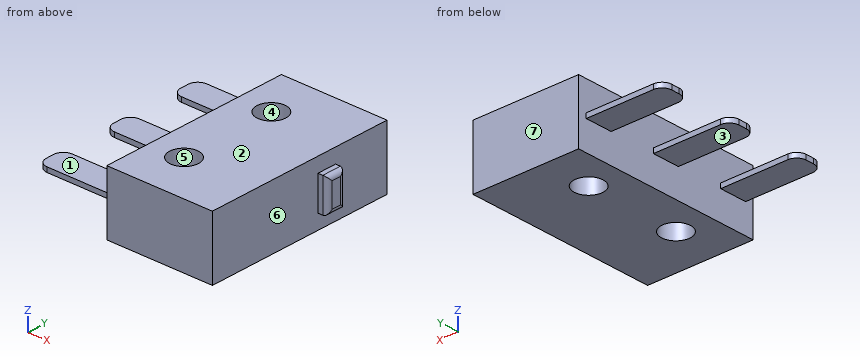
```python
from build123d import *

# Parameters (mm, degrees)
SKETCH_W     = 11
SKETCH_H     = 20
PAD_DEPTH    = 6.5
SKETCH001_W  = 2.85
SKETCH001_H  = 0.5
PAD001_DEPTH = 8
FILLET_R     = 1
SKETCH002_W  = 2
SKETCH002_H  = 3.5
PAD002_DEPTH = 1
FILLET001_R  = 0.5
SKETCH003_R  = 1.5
POCKET_DEPTH = 6.501


with BuildPart() as part:
    # Sketch → Pad (new body)
    with BuildSketch(Plane.XY):
        Rectangle(SKETCH_W, SKETCH_H)
    extrude(amount=PAD_DEPTH)

    # Sketch001 → Pad001 (new body)
    with BuildSketch(Plane(origin=(-5.5, 0, 0), x_dir=(0, -1, 0), z_dir=(-1, 0, 0))):
        with Locations((-7.7, 3.25)):
            Rectangle(SKETCH001_W, SKETCH001_H)
        with Locations((0, 3.25)):
            Rectangle(SKETCH001_W, SKETCH001_H)
        with Locations((7.7, 3.25)):
            Rectangle(SKETCH001_W, SKETCH001_H)
    extrude(amount=PAD001_DEPTH)

    # Fillet
    fillet_edges = [part.edges().sort_by_distance(p)[0] for p in [
        (-13.5, -6.275, 3.25),
        (-13.5, -9.125, 3.25),
        (-13.5, -1.425, 3.25),
        (-13.5, 1.425, 3.25),
        (-13.5, 6.275, 3.25),
        (-13.5, 9.125, 3.25),
    ]]
    fillet(fillet_edges, radius=FILLET_R)

    # Sketch002 → Pad002 (new body)
    with BuildSketch(Plane.YZ.offset(5.5)):
        with Locations((3.1, 3.25)):
            Rectangle(SKETCH002_W, SKETCH002_H)
    extrude(amount=PAD002_DEPTH)

    # Fillet001
    fillet001_edges = [part.edges().sort_by_distance(p)[0] for p in [
        (6.5, 3.1, 5),
        (6.5, 4.1, 3.25),
        (6.5, 3.1, 1.5),
        (6.5, 2.1, 3.25),
    ]]
    fillet(fillet001_edges, radius=FILLET001_R)

    # Sketch003 → Pocket (cut, through all)
    with BuildSketch(Plane(origin=(0, 0, 0), x_dir=(1, 0, 0), z_dir=(0, 0, -1))):
        with Locations((-2, 5)):
            Circle(SKETCH003_R)
        with Locations((-2, -5)):
            Circle(SKETCH003_R)
    extrude(amount=-POCKET_DEPTH, mode=Mode.SUBTRACT)


solid = part.part
```
Verification items for the finished model (mm, model axes). Face numbers are marked on the shaded views. A direction names the side the tool comes from. Coordinates: 2 decimals unless noted, no trailing zeros. Loops run counter-clockwise (first coordinate to the right, second up) from the corner with the lowest first, then second, coordinate; pieces in that order, holes last. Notation, with made-up numbers: (39.5, 37.25) -> (93.5, 37.25) arc R22 cw to (93.5, 44.25) -> close; hole circle Ø1 at (7.5, -36.5). An arc over 180 degrees is marked (long way). Answer in a Markdown table with one row per item. Add a question column.
1. Depth check by flat-ended pin: P1, Ø3, axis at x = -9, y = -8.5, coming from the -Z side; P2, Ø2, axis at y = -2.5, z = 2.5, coming from the -X side; P3, Ø1.4, axis at x = -8, y = 0.5, coming from the +Z side. Enter the tip coordinate at first touch or a pass-through.
2. Draft check along Y on the marked faces 4, 5, 6 and 7. Enter one of: +Y half, -Y half, draft (parallel to the pull), parting line (faces both ways), or undercut.
3. Access from +Z, -Z, +X, -X, +Y, -Y to the whole of each face (thin tool, end or side, straight path). Record for the marked faces 1, 2 and 3.
4. Section check C-C, the plane z = 3.75. Enter the section's corners in (x, y), then the cut area to 3 significant figures.
5. Section check B-B, the plane y = 5. Enter the section's corners in (x, z), then the cut area to 3 significant figures.
6. Material ranges on probe 1 along Y at (x, z) = (-2, 1.5); probe 2 along X at (y, z) = (-5, 2); probe 3 along Y at (x, z) = (-3.25, 2.5), recorded low to high. Write a range as [from, to].
7. Section check A-A, the plane x = -6. Enter the section's corners in (y, z) (3 decimals).
8. Section check D-D, the plane x = -2. Enter the section's corners in (y, z).
Derived:
| question | item | result |
|---|---|---|
| 1 | P1 | stops at z = 3 |
| 1 | P2 | stops at x = -5.5 |
| 1 | P3 | stops at z = 3.5 |
| 2 | face 4 | undercut |
| 2 | face 5 | undercut |
| 2 | face 6 | draft |
| 2 | face 7 | +Y half |
| 3 | face 1 | +Z, -X, +Y, -Y |
| 3 | face 2 | +Z, +X, -X, +Y, -Y |
| 3 | face 3 | -Z, -X, +Y, -Y |
| 4 | outline | (-5.5, -10) -> (5.5, -10) -> (5.5, 2.1) -> (6, 2.1) arc R0.5 ccw to (6.5, 2.6) -> (6.5, 3.6) arc R0.5 ccw to (6, 4.1) -> (5.5, 4.1) -> (5.5, 10) -> (-5.5, 10) -> close; hole circle Ø3 at (-2, -5); hole circle Ø3 at (-2, 5) |
| 4 | area | 208 mm² |
| 5 | outline | (-5.5, 0) -> (-3.5, 0) -> (-3.5, 6.5) -> (-5.5, 6.5) -> close; (-0.5, 0) -> (5.5, 0) -> (5.5, 6.5) -> (-0.5, 6.5) -> close |
| 5 | area | 52.0 mm² |
| 6 | probe 1 | y = [-10, -6.5], [-3.5, 3.5], [6.5, 10] |
| 6 | probe 2 | x = [-5.5, -3.5], [-0.5, 5.5] |
| 6 | probe 3 | y = [-10, -5.83], [-4.17, 4.17], [5.83, 10] |
| 7 | outline | (-9.125, 3) -> (-6.275, 3) -> (-6.275, 3.5) -> (-9.125, 3.5) -> close; (-1.425, 3) -> (1.425, 3) -> (1.425, 3.5) -> (-1.425, 3.5) -> close; (6.275, 3) -> (9.125, 3) -> (9.125, 3.5) -> (6.275, 3.5) -> close |
| 8 | outline | (-10, 0) -> (-6.5, 0) -> (-6.5, 6.5) -> (-10, 6.5) -> close; (-3.5, 0) -> (3.5, 0) -> (3.5, 6.5) -> (-3.5, 6.5) -> close; (6.5, 0) -> (10, 0) -> (10, 6.5) -> (6.5, 6.5) -> close |
